Could you check a few things on this model? Use its own coordinates, in mm. Give positions to 0.01 mm unless a question says otherwise; leave off trailing zeros. Write each loop counter-clockwise with the first axis right and the second up, starting at its lowest first coordinate (ties: lowest second). Pieces come first, ordered by that corner, then holes. Notation, with made-up numbers: (-38, 64.5) - (8, 64.5) arc R13 cw to (8, 80.5) - close; hole circle Ø1 at (-26.5, 50.5). An arc over 180 degrees is marked (long way). Answer as CSV lines item,"result". Start each with the question number.
Q1. We'd pull the mould along X, two halves only. Please class faces 1 (the face through (-168.99, 76.9, 2.46)), 2 (the face through (-167, 118, 0)), 3 (the face through (-165.05, 73.587, 2.465)), 4 (the face through (-175.418, 117.178, 2.465)): pulls with the +X half, pulls with the -X half, needs draft (parallel to the pull), parting line crosses it, or undercut.
Q2. Imagine slicing it at D-D on x = -173.75. List the corners of the cut face in (y, z) for me, and give its area (3 significant figures).
Q3. Imagine slicing it at A-A on x = -165.5. List the corners of the cut face in (y, z) for me, and give its area (3 significant figures).
Q4. Imagine slicing it at C-C on y = 96. List the corners of the cut face in (x, z) for me, and give its area (3 significant figures).
Q5. Will these pins go through, and if not, where does the flat tip stop? pin 1 Ø3 at (x, z) = (-164.5, 2.5) entering from -Y; pin 2 Ø12 at (x, y) = (-159, 95) entering from +Z; pin 3 Ø3 at (x, z) = (-167, 1) entering from +Y; pin 4 Ø1 at (y, z) = (88.5, 4) entering from +X.
Q6. If I drill on line 1 along X through (y, z) = (79, 1.6); line 2 along X through (y, z) = (105.5, 3.5); line 3 along X through (y, z) = (144.5, 0.8), over which ranges is the centre line in solid material (lowest first)?
Q7. Imagine slicing it at B-B on z = 1.9. List the corners of the cut face in (x, y) for me, and give its area (3 significant figures).
Autodesk Inventor part; units mm, degrees
ref_plane "YZ Plane" through (0, 0, 0) normal (1, 0, 0) x (0, 1, 0)
ref_plane "XZ Plane" through (0, 0, 0) normal (0, 1, 0) x (-1, 0, 0)
ref_plane "XY Plane" through (0, 0, 0) normal (0, 0, 1) x (1, 0, 0)
sketch "Sketch1" plane through (0, 0, 0) normal (0, 0, 1) x (1, 0, 0)
  arc A0 (-154.1048, 152.1451) -> (-166.8784, 78.2408) centre (-96.4886, 104.1307) ccw construction
  arc A1 (-157.9458, 155.346) -> (-171.571, 76.5148) centre (-96.4886, 104.1307) ccw
  arc A2 (-150.2637, 148.9441) -> (-162.1857, 79.9668) centre (-96.4886, 104.1307) ccw
  arc A3 (-150.2637, 148.9441) -> (-157.9458, 155.346) centre (-154.1048, 152.1451) ccw
  arc A4 (-171.571, 76.5148) -> (-162.1857, 79.9668) centre (-166.8784, 78.2408) ccw
  line L0 (-154.1048, 152.1451) -> (-96.4886, 104.1307) construction
  line L1 (-96.4886, 104.1307) -> (-166.8784, 78.2408) construction
  point P0 (0, 0)
  dimension "d1" = 75
  dimension "d2" = 10
  dimension "d5" = 60
extrude "Extrusion1" add sketch "Sketch1" along normal blind 5
sketch "Sketch2" plane through (0, 0, 5) normal (0, 0, 1) x (1, 0, 0)
  arc A0 (-157.9458, 155.346) -> (-171.571, 76.5148) centre (-96.4886, 104.1307) ccw
  arc A1 (-171.571, 76.5148) -> (-162.1857, 79.9668) centre (-166.8784, 78.2408) ccw
  arc A2 (-150.2637, 148.9441) -> (-162.1857, 79.9668) centre (-96.4886, 104.1307) ccw
  arc A3 (-150.2637, 148.9441) -> (-157.9458, 155.346) centre (-154.1048, 152.1451) ccw
  point P0 (0, 0)
hole "Hole1" at (-154.1048, 152.1451, 5) at (-166.8784, 78.2408, 5) direction (0, 0, -1) diameter 5 end through all
properties part number "ledeplate"
Conclusion:
1,face 1,"undercut"
1,face 2,"needs draft"
1,face 3,"parting line crosses it"
1,face 4,"pulls with the -X half"
2,outline,"(83.38, 0) - (124.88, 0) - (124.88, 5) - (83.38, 5) - close"
2,area,"208 mm^2"
3,outline,"(73.43, 0) - (76.16, 0) - (76.16, 5) - (73.43, 5) - close; (80.33, 0) - (92.41, 0) - (92.41, 5) - (80.33, 5) - close; (115.85, 0) - (144.6, 0) - (144.6, 5) - (115.85, 5) - close"
3,area,"218 mm^2"
4,outline,"(-176.07, 0) - (-166.01, 0) - (-166.01, 5) - (-176.07, 5) - close"
4,area,"50.3 mm^2"
5,pin 1,"y = 73.32"
5,pin 2,"through"
5,pin 3,"y = 144.6"
5,pin 4,"x = -164.6"
6,line 1,"-172.44 to -169.26, -164.5 to -161.94"
6,line 2,"-176.48 to -166.48"
6,line 3,"-165.56 to -153.68"
7,outline,"(-171.57, 76.51) arc R5 ccw to (-162.19, 79.97) arc R70 cw to (-150.26, 148.94) arc R5 ccw to (-157.95, 155.35) arc R80 ccw to start; hole circle Ø5 at (-166.88, 78.24); hole circle Ø5 at (-154.1, 152.15)"
7,area,"825 mm^2"
